Check sheet for the modelled part. Datum: model origin and axes. Units: mm. A direction names the side the tool comes from. Round coordinates to 2 decimals unless told otherwise and drop trailing zeros. Loops run counter-clockwise (first coordinate to the right, second up) from the corner with the lowest first, then second, coordinate; pieces in that order, holes last. Notation, with made-up numbers: (34, -36.5) -> (80, -36.5) arc R17 ccw to (80, -7.5) -> close; hole circle Ø7 at (-8.5, 69.25). An arc over 180 degrees is marked (long way). Use one line per item in the form item = value. Start each with the question number.
(1) Sectioned sample at A-A (x = 0). Record the cut outline in (y, z), and give its area (3 significant figures).
(2) Material ranges on probe 1 along Y at (x, z) = (-13.75, 0.9); probe 2 along Y at (x, z) = (13.75, 0.7); probe 3 along X at (y, z) = (-23, 1.5), recorded low to high. Write a range as [from, to].
(3) Sectioned sample at D-D (x = 28). Record the cut outline in (y, z), and give its area (3 significant figures).
(4) Sectioned sample at B-B (z = 1.3). State how many separate pieces and enclosed holes the cut face has, and give its area (3 significant figures).
(5) Sectioned sample at C-C (y = 8.8). Record the cut outline in (x, z), and give its area (3 significant figures).
(6) Go/stop test with flat-tipped pins: pin 1 (7.5 mm diameter, centred on x = 13.75, y = 20.15, fed in from -Z); pin 2 (4.5 mm diameter, centred on x = 13.75, y = -19.7, fed in from +Z). Record where each tip stops, or that it passes through.
(7) Draft check along X on faces 1 (the flat face through (10, 0, 4)), 2 (the cylindrical face through (-14.184, -21.652, 2.986)). Enter one of: released by +X, released by -X, zero draft, split by the parting line, or undercut.
(8) Set-up check for faces 3 (the flat face through (16, 19, 2)), 4 (the cylindrical face through (-14.01, 22.133, 2.986)): record each of +Z, -Z, +X, -X, +Y, -Y from which the full face is reachable in a straight line by a thin tool's end or side.
from build123d import *

# Parameters (mm, degrees)
SKETCH1_W           = 60
SKETCH1_H           = 58
SKETCH1_R           = 4.2
SKETCH1_R_2         = 9.6
BOSS_EXTRUDE1_DEPTH = 2
SKETCH4_W           = 60
SKETCH4_H           = 58
SKETCH4_R           = 2
SKETCH4_R_2         = 9.6
BOSS_EXTRUDE3_DEPTH = 2
SKETCH5_R           = 3
CUT_EXTRUDE1_DEPTH  = 4


with BuildPart() as part:
    # Sketch1 → Boss-Extrude1 (new body)
    with BuildSketch(Plane.XY):
        with Locations((10, 0)):
            Rectangle(SKETCH1_W, SKETCH1_H)
        with Locations((13.75, 20.15)):
            Circle(SKETCH1_R, mode=Mode.SUBTRACT)
        with Locations((-13.75, -19.7)):
            Circle(SKETCH1_R, mode=Mode.SUBTRACT)
        with Locations((-5.725, -6.1)):
            Circle(SKETCH1_R, mode=Mode.SUBTRACT)
        with Locations((5.725, -6.1)):
            Circle(SKETCH1_R, mode=Mode.SUBTRACT)
        with BuildLine():
            ThreePointArc((16.186, -16.278610808), (17.171389192, -22.136), (11.314, -23.121389192))
            Line((11.314, -23.121389192), (7.240917629, -20.221389192))
            ThreePointArc((7.240917629, -20.221389192), (6.255528438, -14.364), (12.112917629, -13.378610808))
            Line((12.112917629, -13.378610808), (16.186, -16.278610808))
        make_face(mode=Mode.SUBTRACT)
        with Locations((0, 8.8)):
            Circle(SKETCH1_R_2, mode=Mode.SUBTRACT)
        with Locations((-13.75, 20.15)):
            Circle(SKETCH1_R, mode=Mode.SUBTRACT)
    extrude(amount=BOSS_EXTRUDE1_DEPTH)

    # Sketch4 → Boss-Extrude3 (add)
    with BuildSketch(Plane.XY.offset(2)):
        with Locations((10, 0)):
            Rectangle(SKETCH4_W, SKETCH4_H)
        with Locations((-13.75, -19.7)):
            Circle(SKETCH4_R, mode=Mode.SUBTRACT)
        with Locations((-13.75, 20.15)):
            Circle(SKETCH4_R, mode=Mode.SUBTRACT)
        with Locations((13.75, 20.15)):
            Circle(SKETCH4_R, mode=Mode.SUBTRACT)
        with Locations((13.75, -19.7)):
            Circle(SKETCH4_R, mode=Mode.SUBTRACT)
        with Locations((0, 8.8)):
            Circle(SKETCH4_R_2, mode=Mode.SUBTRACT)
    extrude(amount=BOSS_EXTRUDE3_DEPTH)

    # Sketch5 → Cut-Extrude1 (cut)
    with BuildSketch(Plane.XY.offset(4)):
        with Locations((28, 15)):
            Circle(SKETCH5_R)
        with Locations((28, -15)):
            Circle(SKETCH5_R)
    extrude(amount=-CUT_EXTRUDE1_DEPTH, mode=Mode.SUBTRACT)


solid = part.part
Checks:
q1.outline = (-29, 0) -> (-0.8, 0) -> (-0.8, 4) -> (-29, 4) -> close; (18.4, 0) -> (29, 0) -> (29, 4) -> (18.4, 4) -> close
q1.area = 155 mm2
q2.probe_1 = [-29, -23.9], [-15.5, 15.95], [24.35, 29]
q2.probe_2 = [-29, -23.9], [-14.54, 15.95], [24.35, 29]
q2.probe_3 = [-20, -16.35], [-11.15, 11.14], [16.35, 40]
q3.outline = (-29, 0) -> (-18, 0) -> (-18, 4) -> (-29, 4) -> close; (-12, 0) -> (12, 0) -> (12, 4) -> (-12, 4) -> close; (18, 0) -> (29, 0) -> (29, 4) -> (18, 4) -> close
q3.area = 184 mm2
q4.separate_pieces = 1
q4.enclosed_holes = 9
q4.area = 2,760 mm2
q5.outline = (-20, 0) -> (-9.6, 0) -> (-9.6, 4) -> (-20, 4) -> close; (9.6, 0) -> (40, 0) -> (40, 4) -> (9.6, 4) -> close
q5.area = 163 mm2
q6.pin_1 = 2
q6.pin_2 = 4
q7.face_1 = zero draft
q7.face_2 = undercut
q8.face_3 = -Z
q8.face_4 = +Z, -Z
